from build123d import *

# Parameters (mm, degrees)
SKETCH1_R           = 13
BOSS_EXTRUDE1_DEPTH = 2
CUT_EXTRUDE1_DEPTH  = 2
CUT_EXTRUDE2_DEPTH  = 2


with BuildPart() as part:
    # Sketch1 → Boss-Extrude1 (new body)
    with BuildSketch(Plane.XY):
        Circle(SKETCH1_R)
    extrude(amount=BOSS_EXTRUDE1_DEPTH)

    # Sketch2 → Cut-Extrude1 (cut)
    with BuildSketch(Plane.XY.offset(2)):
        with BuildLine():
            Line((1.85, 2.101784956), (1.85, -2.101784956))
            ThreePointArc((1.85, -2.101784956), (0, -2.8), (-1.85, -2.101784956))
            Line((-1.85, -2.101784956), (-1.85, 2.101784956))
            ThreePointArc((-1.85, 2.101784956), (0, 2.8), (1.85, 2.101784956))
        make_face()
    extrude(amount=-CUT_EXTRUDE1_DEPTH, mode=Mode.SUBTRACT)

    # Sketch3 → Cut-Extrude2 (cut)
    with BuildSketch(Plane.XY.offset(2)):
        with BuildLine():
            Line((-0.344370627, 6.8), (0.344370627, 6.8))
            Line((0.344370627, 6.8), (0.881305494, 11.975564171))
            add(Edge.make_bspline(
                [(-0.881305494, 11.975564171), (0, 12.13877285), (0.881305494, 11.975564171)],
                knots=[0, 0, 0, 1, 1, 1], degree=2))
            Line((-0.881305494, 11.975564171), (-0.344370627, 6.8))
        make_face()
        with BuildLine():
            Line((2.09260599, 6.479165942), (3.950779821, 11.339408071))
            add(Edge.make_bspline(
                [(2.248228346, 11.795605364), (3.141745598, 11.725154195), (3.950779821, 11.339408071)],
                knots=[0, 0, 0, 1, 1, 1], degree=2))
            Line((2.248228346, 11.795605364), (1.427333024, 6.657425296))
            Line((1.427333024, 6.657425296), (2.09260599, 6.479165942))
        make_face()
        with BuildLine():
            Line((3.698233712, 5.716787432), (6.751015032, 9.93049005))
            add(Edge.make_bspline(
                [(5.224549139, 10.811795544), (6.069386425, 10.512485659), (6.751015032, 9.93049005)],
                knots=[0, 0, 0, 1, 1, 1], degree=2))
            Line((5.224549139, 10.811795544), (3.101766288, 6.061158059))
            Line((3.101766288, 6.061158059), (3.698233712, 5.716787432))
        make_face()
        with BuildLine():
            Line((5.051832918, 4.564819306), (9.091179725, 7.844825543))
            add(Edge.make_bspline(
                [(7.844825543, 9.091179725), (8.583408597, 8.583408597), (9.091179725, 7.844825543)],
                knots=[0, 0, 0, 1, 1, 1], degree=2))
            Line((7.844825543, 9.091179725), (4.564819306, 5.051832918))
            Line((4.564819306, 5.051832918), (5.051832918, 4.564819306))
        make_face()
        with BuildLine():
            Line((6.061158059, 3.101766288), (10.811795544, 5.224549139))
            add(Edge.make_bspline(
                [(9.93049005, 6.751015032), (10.512485659, 6.069386425), (10.811795544, 5.224549139)],
                knots=[0, 0, 0, 1, 1, 1], degree=2))
            Line((9.93049005, 6.751015032), (5.716787432, 3.698233712))
            Line((5.716787432, 3.698233712), (6.061158059, 3.101766288))
        make_face()
        with BuildLine():
            Line((6.657425296, 1.427333024), (11.795605364, 2.248228346))
            add(Edge.make_bspline(
                [(11.339408071, 3.950779821), (11.725154195, 3.141745598), (11.795605364, 2.248228346)],
                knots=[0, 0, 0, 1, 1, 1], degree=2))
            Line((11.339408071, 3.950779821), (6.479165942, 2.09260599))
            Line((6.479165942, 2.09260599), (6.657425296, 1.427333024))
        make_face()
        with BuildLine():
            Line((6.8, -0.344370627), (11.975564171, -0.881305494))
            add(Edge.make_bspline(
                [(11.975564171, 0.881305494), (12.13877285, 0), (11.975564171, -0.881305494)],
                knots=[0, 0, 0, 1, 1, 1], degree=2))
            Line((11.975564171, 0.881305494), (6.8, 0.344370627))
            Line((6.8, 0.344370627), (6.8, -0.344370627))
        make_face()
        with BuildLine():
            Line((6.479165942, -2.09260599), (11.339408071, -3.950779821))
            add(Edge.make_bspline(
                [(11.795605364, -2.248228346), (11.725154195, -3.141745598), (11.339408071, -3.950779821)],
                knots=[0, 0, 0, 1, 1, 1], degree=2))
            Line((11.795605364, -2.248228346), (6.657425296, -1.427333024))
            Line((6.657425296, -1.427333024), (6.479165942, -2.09260599))
        make_face()
        with BuildLine():
            Line((5.716787432, -3.698233712), (9.93049005, -6.751015032))
            add(Edge.make_bspline(
                [(10.811795544, -5.224549139), (10.512485659, -6.069386425), (9.93049005, -6.751015032)],
                knots=[0, 0, 0, 1, 1, 1], degree=2))
            Line((10.811795544, -5.224549139), (6.061158059, -3.101766288))
            Line((6.061158059, -3.101766288), (5.716787432, -3.698233712))
        make_face()
        with BuildLine():
            Line((4.564819306, -5.051832918), (7.844825543, -9.091179725))
            add(Edge.make_bspline(
                [(9.091179725, -7.844825543), (8.583408597, -8.583408597), (7.844825543, -9.091179725)],
                knots=[0, 0, 0, 1, 1, 1], degree=2))
            Line((9.091179725, -7.844825543), (5.051832918, -4.564819306))
            Line((5.051832918, -4.564819306), (4.564819306, -5.051832918))
        make_face()
        with BuildLine():
            Line((3.101766288, -6.061158059), (5.224549139, -10.811795544))
            add(Edge.make_bspline(
                [(6.751015032, -9.93049005), (6.069386425, -10.512485659), (5.224549139, -10.811795544)],
                knots=[0, 0, 0, 1, 1, 1], degree=2))
            Line((6.751015032, -9.93049005), (3.698233712, -5.716787432))
            Line((3.698233712, -5.716787432), (3.101766288, -6.061158059))
        make_face()
        with BuildLine():
            Line((1.427333024, -6.657425296), (2.248228346, -11.795605364))
            add(Edge.make_bspline(
                [(3.950779821, -11.339408071), (3.141745598, -11.725154195), (2.248228346, -11.795605364)],
                knots=[0, 0, 0, 1, 1, 1], degree=2))
            Line((3.950779821, -11.339408071), (2.09260599, -6.479165942))
            Line((2.09260599, -6.479165942), (1.427333024, -6.657425296))
        make_face()
        with BuildLine():
            Line((-0.344370627, -6.8), (-0.881305494, -11.975564171))
            add(Edge.make_bspline(
                [(0.881305494, -11.975564171), (0, -12.13877285), (-0.881305494, -11.975564171)],
                knots=[0, 0, 0, 1, 1, 1], degree=2))
            Line((0.881305494, -11.975564171), (0.344370627, -6.8))
            Line((0.344370627, -6.8), (-0.344370627, -6.8))
        make_face()
        with BuildLine():
            Line((-2.09260599, -6.479165942), (-3.950779821, -11.339408071))
            add(Edge.make_bspline(
                [(-2.248228346, -11.795605364), (-3.141745598, -11.725154195), (-3.950779821, -11.339408071)],
                knots=[0, 0, 0, 1, 1, 1], degree=2))
            Line((-2.248228346, -11.795605364), (-1.427333024, -6.657425296))
            Line((-1.427333024, -6.657425296), (-2.09260599, -6.479165942))
        make_face()
        with BuildLine():
            Line((-3.698233712, -5.716787432), (-6.751015032, -9.93049005))
            add(Edge.make_bspline(
                [(-5.224549139, -10.811795544), (-6.069386425, -10.512485659), (-6.751015032, -9.93049005)],
                knots=[0, 0, 0, 1, 1, 1], degree=2))
            Line((-5.224549139, -10.811795544), (-3.101766288, -6.061158059))
            Line((-3.101766288, -6.061158059), (-3.698233712, -5.716787432))
        make_face()
        with BuildLine():
            Line((-5.051832918, -4.564819306), (-9.091179725, -7.844825543))
            add(Edge.make_bspline(
                [(-7.844825543, -9.091179725), (-8.583408597, -8.583408597), (-9.091179725, -7.844825543)],
                knots=[0, 0, 0, 1, 1, 1], degree=2))
            Line((-7.844825543, -9.091179725), (-4.564819306, -5.051832918))
            Line((-4.564819306, -5.051832918), (-5.051832918, -4.564819306))
        make_face()
        with BuildLine():
            Line((-6.061158059, -3.101766288), (-10.811795544, -5.224549139))
            add(Edge.make_bspline(
                [(-9.93049005, -6.751015032), (-10.512485659, -6.069386425), (-10.811795544, -5.224549139)],
                knots=[0, 0, 0, 1, 1, 1], degree=2))
            Line((-9.93049005, -6.751015032), (-5.716787432, -3.698233712))
            Line((-5.716787432, -3.698233712), (-6.061158059, -3.101766288))
        make_face()
        with BuildLine():
            Line((-6.657425296, -1.427333024), (-11.795605364, -2.248228346))
            add(Edge.make_bspline(
                [(-11.339408071, -3.950779821), (-11.725154195, -3.141745598), (-11.795605364, -2.248228346)],
                knots=[0, 0, 0, 1, 1, 1], degree=2))
            Line((-11.339408071, -3.950779821), (-6.479165942, -2.09260599))
            Line((-6.479165942, -2.09260599), (-6.657425296, -1.427333024))
        make_face()
        with BuildLine():
            Line((-6.8, 0.344370627), (-11.975564171, 0.881305494))
            add(Edge.make_bspline(
                [(-11.975564171, -0.881305494), (-12.13877285, 0), (-11.975564171, 0.881305494)],
                knots=[0, 0, 0, 1, 1, 1], degree=2))
            Line((-11.975564171, -0.881305494), (-6.8, -0.344370627))
            Line((-6.8, -0.344370627), (-6.8, 0.344370627))
        make_face()
        with BuildLine():
            Line((-6.479165942, 2.09260599), (-11.339408071, 3.950779821))
            add(Edge.make_bspline(
                [(-11.795605364, 2.248228346), (-11.725154195, 3.141745598), (-11.339408071, 3.950779821)],
                knots=[0, 0, 0, 1, 1, 1], degree=2))
            Line((-11.795605364, 2.248228346), (-6.657425296, 1.427333024))
            Line((-6.657425296, 1.427333024), (-6.479165942, 2.09260599))
        make_face()
        with BuildLine():
            Line((-5.716787432, 3.698233712), (-9.93049005, 6.751015032))
            add(Edge.make_bspline(
                [(-10.811795544, 5.224549139), (-10.512485659, 6.069386425), (-9.93049005, 6.751015032)],
                knots=[0, 0, 0, 1, 1, 1], degree=2))
            Line((-10.811795544, 5.224549139), (-6.061158059, 3.101766288))
            Line((-6.061158059, 3.101766288), (-5.716787432, 3.698233712))
        make_face()
        with BuildLine():
            Line((-4.564819306, 5.051832918), (-7.844825543, 9.091179725))
            add(Edge.make_bspline(
                [(-9.091179725, 7.844825543), (-8.583408597, 8.583408597), (-7.844825543, 9.091179725)],
                knots=[0, 0, 0, 1, 1, 1], degree=2))
            Line((-9.091179725, 7.844825543), (-5.051832918, 4.564819306))
            Line((-5.051832918, 4.564819306), (-4.564819306, 5.051832918))
        make_face()
        with BuildLine():
            Line((-3.101766288, 6.061158059), (-5.224549139, 10.811795544))
            add(Edge.make_bspline(
                [(-6.751015032, 9.93049005), (-6.069386425, 10.512485659), (-5.224549139, 10.811795544)],
                knots=[0, 0, 0, 1, 1, 1], degree=2))
            Line((-6.751015032, 9.93049005), (-3.698233712, 5.716787432))
            Line((-3.698233712, 5.716787432), (-3.101766288, 6.061158059))
        make_face()
        with BuildLine():
            Line((-1.427333024, 6.657425296), (-2.248228346, 11.795605364))
            add(Edge.make_bspline(
                [(-3.950779821, 11.339408071), (-3.141745598, 11.725154195), (-2.248228346, 11.795605364)],
                knots=[0, 0, 0, 1, 1, 1], degree=2))
            Line((-3.950779821, 11.339408071), (-2.09260599, 6.479165942))
            Line((-2.09260599, 6.479165942), (-1.427333024, 6.657425296))
        make_face()
    extrude(amount=-CUT_EXTRUDE2_DEPTH, mode=Mode.SUBTRACT)


solid = part.part
Geometry check sheet. Reference: the model listing, model coordinates, mm. Round coordinates to 2 decimals unless told otherwise and drop trailing zeros. Answer in a Markdown table with one row per item.
(1) Draft check along X on faces 1 (the face through (0, 3, 2)), 2 (the face through (-4.148, 8.403, 1.014)). Enter one of: released by +X, released by -X, zero draft, split by the parting line, or undercut.
Responses:
| item | result |
|---|---|
| face 1 | zero draft |
| face 2 | undercut |
(2) Go/stop test with a flat-tipped pin: P1, Ø1, axis at x = 7, z = 1, coming from the +Y side. Record where the tip stops, or that it passes through.
Responses:
| item | result |
|---|---|
| P1 | stops at y = 11.26 |
(3) Sectioned sample at A-A, the plane x = 7.5. State how many separate pieces and enclosed holes the cut face has, and give its area (3 significant figures).
Responses:
| item | result |
|---|---|
| separate pieces | 8 |
| enclosed holes | 0 |
| area | 23.7 mm² |
(4) Scan lines: probe 1 along Y at (x, z) = (5.5, 0.45); probe 2 along X at (y, z) = (-4.75, 0.6); probe 3 along X at (y, z) = (-4.5, 1.6). Record each from-to range of solid material in increasing order. Write a range as from..to.
Responses:
| item | result |
|---|---|
| probe 1 | y = -11.78..-10.7, -8.2..-6.2, -4.93..4.93, 6.2..8.2, 10.7..11.78 |
| probe 2 | x = -12.1..-9.75, -7.17..-5.28, -4.87..4.87, 5.28..7.17, 9.75..12.1 |
| probe 3 | x = -12.2..-9.19, -6.82..6.82, 9.19..12.2 |
